Can you work these out from the model? Positions are in its coordinate system, mm. A direction names the side the tool comes from. Round coordinates to 2 decimals unless told otherwise and drop trailing zeros. Loops run counter-clockwise (first coordinate to the right, second up) from the corner with the lowest first, then second, coordinate; pieces in that order, holes last. Notation, with made-up numbers: M 80.25,5.5 L 137.25,5.5 A31 ccw 137.25,40.5 Z; hole C 61,-2.5 d5. An arc over 180 degrees is marked long. Answer as CSV lines item,"result".
from build123d import *

# Parameters (mm, degrees)
F0_W     = 120
F0_H     = 50
F1_DEPTH = 75
F2_T     = -2.5
F3_R     = 25
F4_DEPTH = 2.5
F5_W     = 58
F5_H     = 58
F5_R     = 22.5
F6_DEPTH = 2


with BuildPart() as f1:
    # F0 (on Front) → F1 (new body)
    with BuildSketch(Plane.XZ):
        Rectangle(F0_W, F0_H)
    extrude(amount=-F1_DEPTH)

    # F2
    f2_openings = [f1.faces().sort_by_distance(p)[0] for p in [
        (0, 0, 0),
    ]]
    offset(amount=F2_T, openings=f2_openings)

    # F3 (on face) → F4 (cut, through all)
    with BuildSketch(Plane.XY.offset(25)):
        with Locations((0, 44.035366)):
            Circle(F3_R)
    extrude(amount=-F4_DEPTH, mode=Mode.SUBTRACT)

    # F5 (on face) → F6 (join)
    with BuildSketch(Plane.XY.offset(25)):
        with Locations((0, 44.035366)):
            Rectangle(F5_W, F5_H)
        with Locations((0, 44.035366)):
            Circle(F5_R, mode=Mode.SUBTRACT)
    extrude(amount=F6_DEPTH)


solid = f1.part
Item 1: We'd pull the mould along Z, two halves only. Please class faces 1 (the face through (-18, 0, -24)), 2 (the face through (-1, 36, -22.5)), 3 (the face through (-1, 37, -25)): released by +Z, released by -Z, zero draft, split by the parting line, or undercut.
Output:
face 1,"zero draft"
face 2,"undercut"
face 3,"released by -Z"
Item 2: If I drill on line 1 along Z through (x, y) = (36, 16); line 2 along Y through (x, z) = (0, 25.5); line 3 along X through (y, z) = (60, -3.5), over which ranges is the centre line in solid material (lowest first)? Write a range as from..to.
Output:
line 1,"z = -25..-22.5, 22.5..25"
line 2,"y = 15.04..21.54, 66.54..73.04"
line 3,"x = -60..-57.5, 57.5..60"
Item 3: If we section it at B-B on z = 16: Write out the boundary of the cut face in (x, y), then the cut area to 4 significant figures.
Output:
outline,"M -60,0 L -57.5,0 L -57.5,72.5 L 57.5,72.5 L 57.5,0 L 60,0 L 60,75 L -60,75 Z"
area,"662.5 mm2"
Item 4: If we section it at D-D on x = 16.5: Write out the boundary of the cut face in (y, z).
Output:
outline,"M 0,-25 L 75,-25 L 75,25 L 73.04,25 L 73.04,27 L 59.33,27 L 59.33,25 L 62.82,25 L 62.82,22.5 L 72.5,22.5 L 72.5,-22.5 L 0,-22.5 Z; M 0,22.5 L 25.25,22.5 L 25.25,25 L 28.74,25 L 28.74,27 L 15.04,27 L 15.04,25 L 0,25 Z"
Item 5: On a 3-axis mill with a long thin cutter (end or side, diameter ignored), from which of +Z, -Z, +X, -X, +Y, -Y can I reach the whole of each face in a straight line? I mean faces 4 (the face through (-22.34, 47.86, 25)), 5 (the face through (-60, 37, 0)), 6 (the face through (10.382, 24.074, 25.986)), 7 (the face through (-14, 20, 22.5)). Say none if no direction works.
Output:
face 4,"none"
face 5,"+Z, -Z, -X, +Y, -Y"
face 6,"+Z"
face 7,"-Y"
Item 6: If we section it at C-C on x = 41: Write out the boundary of the cut face in (y, z).
Output:
outline,"M 0,-25 L 75,-25 L 75,25 L 0,25 L 0,22.5 L 72.5,22.5 L 72.5,-22.5 L 0,-22.5 Z"
Item 7: If we section it at A-A on x = 0: Write out the boundary of the cut face in (y, z), then the cut area to 4 significant figures.
Output:
outline,"M 0,-25 L 75,-25 L 75,25 L 73.04,25 L 73.04,27 L 66.54,27 L 66.54,25 L 69.04,25 L 69.04,22.5 L 72.5,22.5 L 72.5,-22.5 L 0,-22.5 Z; M 0,22.5 L 19.04,22.5 L 19.04,25 L 21.54,25 L 21.54,27 L 15.04,27 L 15.04,25 L 0,25 Z"
area,"388.5 mm2"
Item 8: Will these pins go through, and if not, where does the flat tip stop? pin 1 (1 mm diameter, centred on x = 5, z = 26, fed in from +Y); pin 2 (1 mm diameter, centred on y = 41, z = 26, fed in from +X); pin 3 (1.5 mm diameter, centred on x = 16.5, y = 34.5, fed in from +Z).
Output:
pin 1,"stops at y = 73.04"
pin 2,"stops at x = 29"
pin 3,"stops at z = -22.5"
